Autodesk Inventor part; units mm, degrees
ref_plane "YZ Plane" through (0, 0, 0) normal (1, 0, 0) x (0, 1, 0)
ref_plane "XZ Plane" through (0, 0, 0) normal (0, 1, 0) x (-1, 0, 0)
ref_plane "XY Plane" through (0, 0, 0) normal (0, 0, 1) x (1, 0, 0)
sketch "Sketch2" plane through (0, 0, 0) normal (0, 1, 0) x (-1, 0, 0)
  line L0 (2.5667, 3.1167) -> (0.5667, 3.1167)
  line L1 (0.5667, 3.1167) -> (0.5667, 1.1167)
  line L2 (0.5667, 1.1167) -> (2.5667, 1.1167)
  line L3 (2.5667, 1.1167) -> (2.5667, 3.1167)
  point P0 (0, 0)
  dimension "d5" = 2
  dimension "d6" = 2
extrude "Extrusion1" add sketch "Sketch2" along normal blind 20
sketch "Sketch3" plane through (-0.5667, 0, 3.1167) normal (1, 0, 0) x (0, 0, -1)
  line L0 (0, 20) -> (2, 20)
  line L1 (0, 20) -> (2, 18)
  line L2 (2, 0) -> (2, 20)
  line L3 (0, 20) -> (2.8284, 20) construction
  point P0 (3.1167, 0)
  dimension "d9" = 45
extrude "Extrusion2" cut sketch "Sketch3" against normal through all
sketch "Sketch4" plane through (0, 0, 0) normal (0, -1, 0) x (1, 0, 0)
  line L0 (3.4333, 7.1167) -> (-6.5667, 7.1167)
  line L1 (-6.5667, 7.1167) -> (-6.5667, -2.8833)
  line L2 (-6.5667, -2.8833) -> (3.4333, -2.8833)
  line L3 (3.4333, -2.8833) -> (3.4333, 7.1167)
  line L4 (-2.5667, 1.1167) -> (-2.5667, 3.1167)
  line L5 (-0.5667, 1.1167) -> (-2.5667, 1.1167)
  point P0 (0, 0)
  dimension "d12" = 10
  dimension "d13" = 10
  dimension "d14" = 4
  dimension "d15" = 4
extrude "Extrusion3" add sketch "Sketch4" along normal blind 1
sketch "Sketch5" plane through (0, 0, 0) normal (0, 1, 0) x (1, 0, 0)
  circle A0 centre (-5.5667, 1.8833) radius 0.25
  line L0 (-6.5667, -7.1167) -> (-6.5667, 2.8833)
  line L1 (3.4333, 2.8833) -> (3.4333, -7.1167)
  line L2 (-6.5667, 2.8833) -> (3.4333, 2.8833)
  circle A1 centre (-5.5667, -6.1167) radius 0.25
  circle A2 centre (2.4333, 1.8833) radius 0.25
  circle A3 centre (2.4333, -6.1167) radius 0.25
  point P0 (0, 0)
  dimension "d18" = 0.5
  dimension "d20" = 9
  dimension "d22" = 1
  dimension "d25" = 8
  dimension "d28" = 8
extrude "Extrusion4" cut sketch "Sketch5" against normal through all
properties part number "Viewing Mirror Holder"
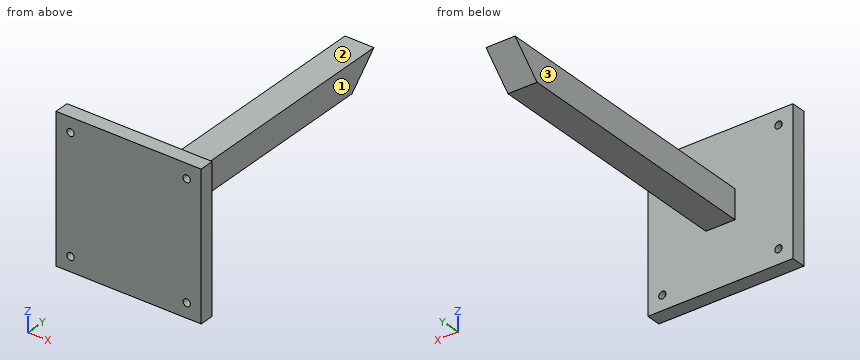
Geometry: final body of the model. Coordinates: model frame, mm. Face numbers are marked on the shaded views. A direction names the side the tool comes from. Coordinates: 2 decimals unless noted, no trailing zeros. Order: outer loops, then holes, each group sorted by start corner. A loop starts at its lowest first (then second) coordinate and runs counter-clockwise, first axis right, second up. Notation, with made-up numbers: (60.25, 29.25) - (84.25, 29.25) arc R9 ccw to (84.25, 43.25) - close; hole circle Ø7 at (9, 44). An arc over 180 degrees is marked (long way). Return JSON: item names as keys, results as strings. Group by question number.
1. Cut plane A-A (z = 2.5). Output: boundary loops of the cut face in (x, y).
2. Set-up query: the marked faces 1, 2 and 3. Return all of +Z, -Z, +X, -X, +Y, -Y with unobstructed straight access to the full face (end or side cutting, diameter ignored); none if empty.
3. Material intervals for line 1 along Y through (x, z) = (0, 1.25); line 2 along X through (y, z) = (4.25, 2.75); line 3 along Z through (x, y) = (-0.75, 10.5), sorted ascending. Write a range as [from, to].
4. Cut plane B-B (y = 5.25). Output: boundary loops of the cut face in (x, z).
5. Pin query (flat end, axial travel): pin 1 (5 mm diameter, centred on y = 15, z = 4.5, fed in from -X); pin 2 (3 mm diameter, centred on x = -4.5, z = 3.5, fed in from +Y); pin 3 (2 mm diameter, centred on x = -1, y = 7.5, fed in from -Z). Return the tip coordinate at first contact, or that it passes through.
6. Cut plane C-C (x = -3.5). Output: boundary loops of the cut face in (y, z).
Resolved:
{
 "1": {"outline": "(-6.57, -1) - (3.43, -1) - (3.43, 0) - (-0.57, 0) - (-0.57, 19.38) - (-2.57, 19.38) - (-2.57, 0) - (-6.57, 0) - close"},
 "2": {"face 1": "+Z, -Z, +X, +Y", "face 2": "+Z, +X, -X, +Y", "face 3": "+Z, -Z, -X, +Y"},
 "3": {"line 1": "y = [-1, 0]", "line 2": "x = [-2.57, -0.57]", "line 3": "z = [1.12, 3.12]"},
 "4": {"outline": "(-2.57, 1.12) - (-0.57, 1.12) - (-0.57, 3.12) - (-2.57, 3.12) - close"},
 "5": {"pin 1": "stops at x = -2.57", "pin 2": "stops at y = 0", "pin 3": "stops at z = 1.12"},
 "6": {"outline": "(-1, -2.88) - (0, -2.88) - (0, 7.12) - (-1, 7.12) - close"}
}
